```python
from build123d import *

# Parameters (mm, degrees)
BOSS_EXTRUDE1_DEPTH        = 10
BOSS_EXTRUDE1_2_DEPTH      = 10
CUT_EXTRUDE1_START         = -3
CUT_EXTRUDE1_DEPTH         = 3
BOSS_EXTRUDE2_DEPTH        = 3
BOSS_EXTRUDE2_DEPTH_BACK   = 3
SKETCH4_R                  = 3
SKETCH4_R_2                = 1.75
BOSS_EXTRUDE2_2_DEPTH      = 3
BOSS_EXTRUDE2_2_DEPTH_BACK = 3
BOSS_EXTRUDE2_3_DEPTH      = 3
BOSS_EXTRUDE2_3_DEPTH_BACK = 3
BOSS_EXTRUDE2_4_DEPTH      = 3
BOSS_EXTRUDE2_4_DEPTH_BACK = 3
BOSS_EXTRUDE3_DEPTH        = 3


with BuildPart() as part:
    # Sketch2 → Boss-Extrude1 (new body)
    with BuildSketch(Plane(origin=(0, 33.1, 0), x_dir=(1, 0, 0), z_dir=(0, 1, 0))):
        with BuildLine():
            ThreePointArc((53.031183993, 11.75), (56.781183993, 15.5), (53.031183993, 19.25))
            Line((53.031183993, 19.25), (-26.968816007, 19.25))
            ThreePointArc((-26.968816007, 19.25), (-30.718816007, 15.5), (-26.968816007, 11.75))
            Line((-26.968816007, 11.75), (53.031183993, 11.75))
        make_face()
        with BuildLine():
            ThreePointArc((-26.968816007, 13.75), (-28.718816007, 15.5), (-26.968816007, 17.25))
            Line((-26.968816007, 17.25), (53.031183993, 17.25))
            ThreePointArc((53.031183993, 17.25), (54.781183993, 15.5), (53.031183993, 13.75))
            Line((53.031183993, 13.75), (-26.968816007, 13.75))
        make_face(mode=Mode.SUBTRACT)
    extrude(amount=BOSS_EXTRUDE1_DEPTH)


with BuildPart() as body_2:
    # Sketch2 → Boss-Extrude1 2 (new body)
    with BuildSketch(Plane(origin=(0, 33.1, 0), x_dir=(1, 0, 0), z_dir=(0, 1, 0))):
        with BuildLine():
            ThreePointArc((-26.968816007, -11.75), (-30.718816007, -15.5), (-26.968816007, -19.25))
            Line((-26.968816007, -19.25), (53.031183993, -19.25))
            ThreePointArc((53.031183993, -19.25), (56.781183993, -15.5), (53.031183993, -11.75))
            Line((53.031183993, -11.75), (-26.968816007, -11.75))
        make_face()
        with BuildLine():
            ThreePointArc((-26.968816007, -17.25), (-28.718816007, -15.5), (-26.968816007, -13.75))
            Line((-26.968816007, -13.75), (53.031183993, -13.75))
            ThreePointArc((53.031183993, -13.75), (54.781183993, -15.5), (53.031183993, -17.25))
            Line((53.031183993, -17.25), (-26.968816007, -17.25))
        make_face(mode=Mode.SUBTRACT)
    extrude(amount=BOSS_EXTRUDE1_2_DEPTH)


with BuildPart() as cut_extrude1_tool:
    # Sketch3 → Cut-Extrude1 (new body)
    with BuildSketch(Plane(origin=(0, 43.1, 0), x_dir=(1, 0, 0), z_dir=(0, 1, 0)).offset(CUT_EXTRUDE1_START)):
        with BuildLine():
            ThreePointArc((-26.968816007, 13.75), (-28.718816007, 15.5), (-26.968816007, 17.25))
            Line((-26.968816007, 17.25), (-24.532117421, 17.25))
            ThreePointArc((-24.532117421, 17.25), (-25.599509613, 18.169269563), (-26.968816007, 18.5))
            ThreePointArc((-26.968816007, 18.5), (-29.968816007, 15.5), (-26.968816007, 12.5))
            ThreePointArc((-26.968816007, 12.5), (-25.599509613, 12.830730437), (-24.532117421, 13.75))
            Line((-24.532117421, 13.75), (-26.968816007, 13.75))
        make_face()
        with BuildLine():
            Line((-24.532117421, 17.25), (-26.968816007, 17.25))
            ThreePointArc((-26.968816007, 17.25), (-28.718816007, 15.5), (-26.968816007, 13.75))
            Line((-26.968816007, 13.75), (-24.532117421, 13.75))
            ThreePointArc((-24.532117421, 13.75), (-24.113111561, 14.580787228), (-23.968816007, 15.5))
            ThreePointArc((-23.968816007, 15.5), (-24.113111561, 16.419212772), (-24.532117421, 17.25))
        make_face()
        with BuildLine():
            ThreePointArc((-26.968816007, 18.5), (-25.599509613, 18.169269563), (-24.532117421, 17.25))
            Line((-24.532117421, 17.25), (50.594485407, 17.25))
            ThreePointArc((50.594485407, 17.25), (51.661877599, 18.169269563), (53.031183993, 18.5))
            Line((53.031183993, 18.5), (-26.968816007, 18.5))
        make_face()
        with BuildLine():
            Line((50.594485407, 13.75), (-24.532117421, 13.75))
            ThreePointArc((-24.532117421, 13.75), (-25.599509613, 12.830730437), (-26.968816007, 12.5))
            Line((-26.968816007, 12.5), (53.031183993, 12.5))
            ThreePointArc((53.031183993, 12.5), (51.661877599, 12.830730437), (50.594485407, 13.75))
        make_face()
        with BuildLine():
            ThreePointArc((53.031183993, 18.5), (51.661877599, 18.169269563), (50.594485407, 17.25))
            Line((50.594485407, 17.25), (53.031183993, 17.25))
            ThreePointArc((53.031183993, 17.25), (54.781183993, 15.5), (53.031183993, 13.75))
            Line((53.031183993, 13.75), (50.594485407, 13.75))
            ThreePointArc((50.594485407, 13.75), (51.661877599, 12.830730437), (53.031183993, 12.5))
            ThreePointArc((53.031183993, 12.5), (55.152504337, 13.378679656), (56.031183993, 15.5))
            ThreePointArc((56.031183993, 15.5), (55.152504337, 17.621320344), (53.031183993, 18.5))
        make_face()
        with BuildLine():
            Line((53.031183993, 17.25), (50.594485407, 17.25))
            ThreePointArc((50.594485407, 17.25), (50.031183993, 15.5), (50.594485407, 13.75))
            Line((50.594485407, 13.75), (53.031183993, 13.75))
            ThreePointArc((53.031183993, 13.75), (54.781183993, 15.5), (53.031183993, 17.25))
        make_face()
        with BuildLine():
            ThreePointArc((-26.968816007, -13.75), (-28.718816007, -15.5), (-26.968816007, -17.25))
            Line((-26.968816007, -17.25), (-24.532117421, -17.25))
            ThreePointArc((-24.532117421, -17.25), (-24.113111561, -16.419212772), (-23.968816007, -15.5))
            ThreePointArc((-23.968816007, -15.5), (-24.113111561, -14.580787228), (-24.532117421, -13.75))
            Line((-24.532117421, -13.75), (-26.968816007, -13.75))
        make_face()
        with BuildLine():
            Line((-24.532117421, -17.25), (-26.968816007, -17.25))
            ThreePointArc((-26.968816007, -17.25), (-28.718816007, -15.5), (-26.968816007, -13.75))
            Line((-26.968816007, -13.75), (-24.532117421, -13.75))
            ThreePointArc((-24.532117421, -13.75), (-25.599509613, -12.830730437), (-26.968816007, -12.5))
            ThreePointArc((-26.968816007, -12.5), (-29.968816007, -15.5), (-26.968816007, -18.5))
            ThreePointArc((-26.968816007, -18.5), (-25.599509613, -18.169269563), (-24.532117421, -17.25))
        make_face()
        with BuildLine():
            ThreePointArc((-26.968816007, -12.5), (-25.599509613, -12.830730437), (-24.532117421, -13.75))
            Line((-24.532117421, -13.75), (50.594485407, -13.75))
            ThreePointArc((50.594485407, -13.75), (51.661877599, -12.830730437), (53.031183993, -12.5))
            Line((53.031183993, -12.5), (-26.968816007, -12.5))
        make_face()
        with BuildLine():
            Line((50.594485407, -17.25), (-24.532117421, -17.25))
            ThreePointArc((-24.532117421, -17.25), (-25.599509613, -18.169269563), (-26.968816007, -18.5))
            Line((-26.968816007, -18.5), (53.031183993, -18.5))
            ThreePointArc((53.031183993, -18.5), (51.661877599, -18.169269563), (50.594485407, -17.25))
        make_face()
        with BuildLine():
            ThreePointArc((50.594485407, -13.75), (50.031183993, -15.5), (50.594485407, -17.25))
            Line((50.594485407, -17.25), (53.031183993, -17.25))
            ThreePointArc((53.031183993, -17.25), (54.781183993, -15.5), (53.031183993, -13.75))
            Line((53.031183993, -13.75), (50.594485407, -13.75))
        make_face()
        with BuildLine():
            Line((53.031183993, -17.25), (50.594485407, -17.25))
            ThreePointArc((50.594485407, -17.25), (51.661877599, -18.169269563), (53.031183993, -18.5))
            ThreePointArc((53.031183993, -18.5), (55.152504337, -17.621320344), (56.031183993, -15.5))
            ThreePointArc((56.031183993, -15.5), (55.152504337, -13.378679656), (53.031183993, -12.5))
            ThreePointArc((53.031183993, -12.5), (51.661877599, -12.830730437), (50.594485407, -13.75))
            Line((50.594485407, -13.75), (53.031183993, -13.75))
            ThreePointArc((53.031183993, -13.75), (54.781183993, -15.5), (53.031183993, -17.25))
        make_face()
    extrude(amount=CUT_EXTRUDE1_DEPTH)


with BuildPart() as part_1:
    add(part.part)

    # Cut-Extrude1: cut by cut_extrude1_tool
    add(cut_extrude1_tool.part, mode=Mode.SUBTRACT)



with BuildPart() as body_2_1:
    add(body_2.part)

    # Cut-Extrude1: cut by cut_extrude1_tool
    add(cut_extrude1_tool.part, mode=Mode.SUBTRACT)


with BuildPart() as body_3:
    # Sketch4 → Boss-Extrude2 (new, two sides: drawn at the far end of the back side and taken through both)
    with BuildSketch(Plane(origin=(0, 43.1, 0), x_dir=(1, 0, 0), z_dir=(0, 1, 0)).offset(-BOSS_EXTRUDE2_DEPTH_BACK)):
        with Locations(Location((-15.968816007, 24.5, 0), (0, 0, 270))):
            Circle(SKETCH4_R)
        with Locations(Location((-15.968816007, 24.5, 0), (0, 0, 270))):
            Circle(SKETCH4_R_2, mode=Mode.SUBTRACT)
    extrude(amount=BOSS_EXTRUDE2_DEPTH + BOSS_EXTRUDE2_DEPTH_BACK)


with BuildPart() as body_4:
    # Sketch4 → Boss-Extrude2 2 (new, two sides: drawn at the far end of the back side and taken through both)
    with BuildSketch(Plane(origin=(0, 43.1, 0), x_dir=(1, 0, 0), z_dir=(0, 1, 0)).offset(-BOSS_EXTRUDE2_2_DEPTH_BACK)):
        with Locations(Location((42.031183993, 24.5, 0), (0, 0, 90))):
            Circle(SKETCH4_R)
        with Locations(Location((42.031183993, 24.5, 0), (0, 0, 90))):
            Circle(SKETCH4_R_2, mode=Mode.SUBTRACT)
    extrude(amount=BOSS_EXTRUDE2_2_DEPTH + BOSS_EXTRUDE2_2_DEPTH_BACK)


with BuildPart() as body_5:
    # Sketch4 → Boss-Extrude2 3 (new, two sides: drawn at the far end of the back side and taken through both)
    with BuildSketch(Plane(origin=(0, 43.1, 0), x_dir=(1, 0, 0), z_dir=(0, 1, 0)).offset(-BOSS_EXTRUDE2_3_DEPTH_BACK)):
        with Locations(Location((42.031183993, -24.5, 0), (0, 0, 270))):
            Circle(SKETCH4_R)
        with Locations(Location((42.031183993, -24.5, 0), (0, 0, 270))):
            Circle(SKETCH4_R_2, mode=Mode.SUBTRACT)
    extrude(amount=BOSS_EXTRUDE2_3_DEPTH + BOSS_EXTRUDE2_3_DEPTH_BACK)


with BuildPart() as body_6:
    # Sketch4 → Boss-Extrude2 4 (new, two sides: drawn at the far end of the back side and taken through both)
    with BuildSketch(Plane(origin=(0, 43.1, 0), x_dir=(1, 0, 0), z_dir=(0, 1, 0)).offset(-BOSS_EXTRUDE2_4_DEPTH_BACK)):
        with Locations(Location((-15.968816007, -24.5, 0), (0, 0, 90))):
            Circle(SKETCH4_R)
        with Locations(Location((-15.968816007, -24.5, 0), (0, 0, 90))):
            Circle(SKETCH4_R_2, mode=Mode.SUBTRACT)
    extrude(amount=BOSS_EXTRUDE2_4_DEPTH + BOSS_EXTRUDE2_4_DEPTH_BACK)


with BuildPart() as part_2:
    add(part_1.part)

    add(body_2_1.part)  # Boss-Extrude3 merges body 2

    add(body_3.part)  # Boss-Extrude3 merges body 3

    add(body_4.part)  # Boss-Extrude3 merges body 4

    add(body_5.part)  # Boss-Extrude3 merges body 5

    add(body_6.part)  # Boss-Extrude3 merges body 6
    # Sketch5 → Boss-Extrude3 (add)
    with BuildSketch(Plane.XZ.offset(-40.1)):
        with BuildLine():
            Line((-14.403158686, -19.25), (-17.904870954, -22.208343123))
            ThreePointArc((-17.904870954, -22.208343123), (-14.705519692, -21.778955638), (-12.968816007, -24.5))
            ThreePointArc((-12.968816007, -24.5), (-13.247771645, -25.763296315), (-14.032761059, -26.791656877))
            Line((-14.032761059, -26.791656877), (-5.105901899, -19.25))
            Line((-5.105901899, -19.25), (-14.403158686, -19.25))
        make_face()
        Polygon((8.3825556, 0), (-5.525607665, -11.75), (3.771649121, -11.75), (13.031183993, -3.927289505), align=None)
        Polygon((13.031183993, 3.927289505), (8.3825556, 0), (13.031183993, -3.927289505), (17.679812386, 0), align=None)
        Polygon((17.679812386, 0), (13.031183993, -3.927289505), (22.290718865, -11.75), (31.587975652, -11.75), align=None)
        with BuildLine():
            Line((40.465526672, -19.25), (31.168269886, -19.25))
            Line((31.168269886, -19.25), (40.095129046, -26.791656877))
            ThreePointArc((40.095129046, -26.791656877), (39.739527117, -22.563945052), (43.967238941, -22.208343123))
            Line((43.967238941, -22.208343123), (40.465526672, -19.25))
        make_face()
        Polygon((-5.525607665, 11.75), (8.3825556, 0), (13.031183993, 3.927289505), (3.771649121, 11.75), align=None)
        with BuildLine():
            Line((-17.904870954, 22.208343123), (-14.403158686, 19.25))
            Line((-14.403158686, 19.25), (-5.105901899, 19.25))
            Line((-5.105901899, 19.25), (-14.032761059, 26.791656877))
            ThreePointArc((-14.032761059, 26.791656877), (-13.247771645, 25.763296315), (-12.968816007, 24.5))
            ThreePointArc((-12.968816007, 24.5), (-14.705519692, 21.778955638), (-17.904870954, 22.208343123))
        make_face()
        Polygon((22.290718865, 11.75), (13.031183993, 3.927289505), (17.679812386, 0), (31.587975652, 11.75), align=None)
        with BuildLine():
            Line((40.095129046, 26.791656877), (31.168269886, 19.25))
            Line((31.168269886, 19.25), (40.465526672, 19.25))
            Line((40.465526672, 19.25), (43.967238941, 22.208343123))
            ThreePointArc((43.967238941, 22.208343123), (39.739527117, 22.563945052), (40.095129046, 26.791656877))
        make_face()
    extrude(amount=-BOSS_EXTRUDE3_DEPTH)


solid = part_2.part
```
The model under review builds one solid part; all positions refer to its coordinate system, in mm. A direction names the side the tool comes from. Round coordinates to 2 decimals unless told otherwise and drop trailing zeros. Order: outer loops, then holes, each group sorted by start corner. A loop starts at its lowest first (then second) coordinate and runs counter-clockwise, first axis right, second up. Notation, with made-up numbers: (-5, 26.25) - (7, 26.25) arc R16 cw to (7, 37.25) - close; hole circle Ø8 at (50.5, 64.25). An arc over 180 degrees is marked (long way). Answer in a Markdown table with one row per item.
(1) Take a section at B-B on y = 44.75. Write out the cut boundary in (x, z), plus the area to 3 significant figures.
Result set:
| item | result |
|---|---|
| outline | circle Ø6 at (-15.97, -24.5); circle Ø6 at (-15.97, 24.5); circle Ø6 at (42.03, -24.5); circle Ø6 at (42.03, 24.5); hole circle Ø3.5 at (-15.97, -24.5); hole circle Ø3.5 at (-15.97, 24.5); hole circle Ø3.5 at (42.03, -24.5); hole circle Ø3.5 at (42.03, 24.5) |
| area | 74.6 mm2 |
(2) Machinability: for faces 1 (the face through (13, 40.1, 0)), 2 (the face through (-14, 46.1, 25)), 3 (the face through (-18.897, 43.725, -25.15)), 4 (the face through (17.726, 41.579, 7.893)), which of the approach directions +Z, -Z, +X, -X, +Y, -Y give a long, thin tool a straight path to every point of the face, cutting with its end or side? Answer none if there is none.
Result set:
| item | result |
|---|---|
| face 1 | +X, -X, -Y |
| face 2 | +Z, -Z, +X, -X, +Y |
| face 3 | +Y |
| face 4 | +Y, -Y |
(3) Take a section at A-A on y = 39. Write out the cut boundary in (x, z), plus the area to 3 significant figures.
Result set:
| item | result |
|---|---|
| outline | (-26.97, -19.25) - (53.03, -19.25) arc R3.75 ccw to (53.03, -11.75) - (-26.97, -11.75) arc R3.75 ccw to start; (-26.97, 11.75) - (53.03, 11.75) arc R3.75 ccw to (53.03, 19.25) - (-26.97, 19.25) arc R3.75 ccw to start; hole (-26.97, -17.25) - (53.03, -17.25) arc R1.75 ccw to (53.03, -13.75) - (-26.97, -13.75) arc R1.75 ccw to start; hole (-26.97, 13.75) - (53.03, 13.75) arc R1.75 ccw to (53.03, 17.25) - (-26.97, 17.25) arc R1.75 ccw to start |
| area | 709 mm2 |
(4) Take a section at C-C on z = 24.5. Write out the cut boundary in (x, y), plus the area to 3 significant figures.
Result set:
| item | result |
|---|---|
| outline | (-18.97, 40.1) - (-17.72, 40.1) - (-17.72, 46.1) - (-18.97, 46.1) - close; (-14.22, 40.1) - (-11.32, 40.1) - (-11.32, 43.1) - (-12.97, 43.1) - (-12.97, 46.1) - (-14.22, 46.1) - close; (37.38, 40.1) - (40.28, 40.1) - (40.28, 46.1) - (39.03, 46.1) - (39.03, 43.1) - (37.38, 43.1) - close; (43.78, 40.1) - (45.03, 40.1) - (45.03, 46.1) - (43.78, 46.1) - close |
| area | 39.9 mm2 |
(5) For line 1 (Z direction, x = 1.5, y = 40); line 2 (X direction, y = 44.05, z = 24.5); line 3 (X direction, y = 43.5, z = 25.5), list the stretches that pass through material, from the lowest coordinate up. Write a range as from..to.
Result set:
| item | result |
|---|---|
| line 1 | z = -19.25..-17.25, -13.75..-11.75, 11.75..13.75, 17.25..19.25 |
| line 2 | x = -18.97..-17.72, -14.22..-12.97, 39.03..40.28, 43.78..45.03 |
| line 3 | x = -18.8..-17.4, -14.53..-13.14, 39.2..40.6, 43.47..44.86 |
(6) Mouldability with a two-part tool opening along Z and no side actions: class faces 5 (the face through (40, 40.1, -22)), 6 (the face through (35.57, 41.58, -22.97)), 7 (the face through (8.47, 41.58, 7.78)) as released by +Z, released by -Z, zero draft, split by the parting line, or undercut.
Result set:
| item | result |
|---|---|
| face 5 | zero draft |
| face 6 | released by -Z |
| face 7 | undercut |
(7) Take a section at D-D on x = -25. Write out the cut boundary in (y, z), plus the area to 3 significant figures.
Result set:
| item | result |
|---|---|
| outline | (33.1, -19.25) - (43.1, -19.25) - (43.1, -18.5) - (40.1, -18.5) - (40.1, -17.25) - (33.1, -17.25) - close; (33.1, -13.75) - (40.1, -13.75) - (40.1, -12.5) - (43.1, -12.5) - (43.1, -11.75) - (33.1, -11.75) - close; (33.1, 11.75) - (43.1, 11.75) - (43.1, 12.5) - (40.1, 12.5) - (40.1, 13.75) - (33.1, 13.75) - close; (33.1, 17.25) - (40.1, 17.25) - (40.1, 18.5) - (43.1, 18.5) - (43.1, 19.25) - (33.1, 19.25) - close |
| area | 65.0 mm2 |
(8) Clearance check with flat-ended pins moving along their axes: P1, Ø3.5, axis at x = 5.5, y = 41, coming from the -Z side; P2, Ø1, axis at y = 43.5, z = -15, coming from the -X side; P3, Ø12, axis at x = 25.5, z = -12.5, coming from the +Y side; P4, Ø3, axis at x = -15.97, z = -24.5, coming from the +Y side. State where each tip first meets the part, or that it passes through.
Result set:
| item | result |
|---|---|
| P1 | stops at z = -19.25 |
| P2 | stops at x = -30.71 |
| P3 | stops at y = 43.1 |
| P4 | passes through |
